Part model, mm, in its own coordinate system. Face numbers are marked on the shaded views. A direction names the side the tool comes from. Coordinates: 2 decimals unless noted, no trailing zeros. Write each loop counter-clockwise with the first axis right and the second up, starting at its lowest first coordinate (ties: lowest second). Pieces come first, ordered by that corner, then holes. Notation, with made-up numbers: (-18, 10.5) - (-5, 10.5) arc R13 cw to (-5, 21.5) - close; hole circle Ø6 at (-32.5, 52). An arc over 180 degrees is marked (long way). Use a Markdown table: item, result.
```python
from build123d import *

# Parameters (mm, degrees)
SKETCH1_W           = 30
SKETCH1_H           = 30
BOSS_EXTRUDE1_DEPTH = 2
SKETCH2_R           = 9
CUT_EXTRUDE1_DEPTH  = 22.307275753
FILLET1_R           = 15
SKETCH3_W           = 30
SKETCH3_H           = 2
BOSS_EXTRUDE2_DEPTH = 11
SKETCH4_R           = 1.5
CUT_EXTRUDE2_DEPTH  = 34.615472628
FILLET2_R           = 2


with BuildPart() as part:
    # Sketch1 → Boss-Extrude1 (new body)
    with BuildSketch(Plane.XY):
        Rectangle(SKETCH1_W, SKETCH1_H)
    extrude(amount=BOSS_EXTRUDE1_DEPTH)

    # Sketch2 → Cut-Extrude1 (cut, through all)
    with BuildSketch(Plane.XY.offset(2)):
        Circle(SKETCH2_R)
    extrude(amount=-CUT_EXTRUDE1_DEPTH, mode=Mode.SUBTRACT)

    # Fillet1
    fillet1_edges = [part.edges().sort_by_distance(p)[0] for p in [
        (-15, 15, 1),
        (15, 15, 1),
    ]]
    fillet(fillet1_edges, radius=FILLET1_R - 0.0001)  # a hair under: the kernel refuses the full size

    # Sketch3 → Boss-Extrude2 (add)
    with BuildSketch(Plane(origin=(0, 0, 0), x_dir=(-1, 0, 0), z_dir=(0, 0, -1))):
        with Locations((0, -14)):
            Rectangle(SKETCH3_W, SKETCH3_H)
    extrude(amount=BOSS_EXTRUDE2_DEPTH)

    # Sketch4 → Cut-Extrude2 (cut, through all)
    with BuildSketch(Plane(origin=(0, -13, 0), x_dir=(1, 0, 0), z_dir=(0, 1, 0))):
        with Locations(Location((0, 6, 0), (0, 0, 270))):
            Circle(SKETCH4_R)
    extrude(amount=-CUT_EXTRUDE2_DEPTH, mode=Mode.SUBTRACT)

    # Fillet2
    fillet2_edges = [part.edges().sort_by_distance(p)[0] for p in [
        (15, -14, -11),
        (-15, -14, -11),
        (0, -15, 2),
    ]]
    fillet(fillet2_edges, radius=FILLET2_R)


solid = part.part
```
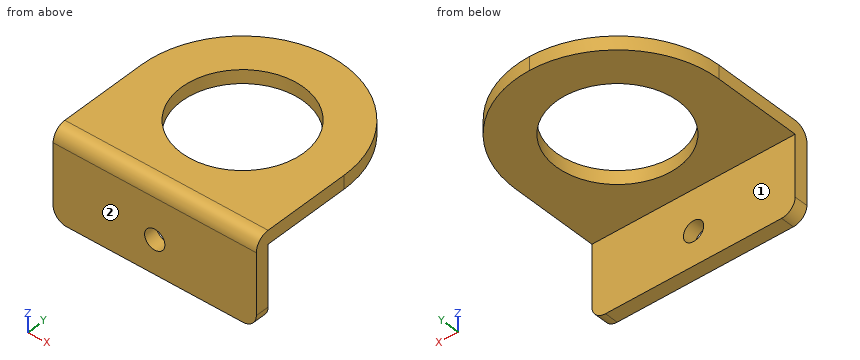
Item 1: Band-saw the part on A-A, the plane z = -6. Give the cut face in (x, y).
From the geometry:
| item | result |
|---|---|
| outline | (-15, -15) - (-1.5, -15) - (-1.5, -13) - (-15, -13) - close; (1.5, -15) - (15, -15) - (15, -13) - (1.5, -13) - close |
Item 2: Which spindle directions (+Z, -Z, +X, -X, +Y, -Y) get a long thin tool onto all of the face, cutting with end or side? Do the marked faces 1 and 2. Say none if no direction does.
From the geometry:
| item | result |
|---|---|
| face 1 | -Z, +X, -X, +Y |
| face 2 | +Z, -Z, +X, -X, -Y |
Item 3: Band-saw the part on B-B, the plane y = -4. Give the cut face in (x, z), then the cut area to 3 significant figures.
From the geometry:
| item | result |
|---|---|
| outline | (-15, 0) - (-8.06, 0) - (-8.06, 2) - (-15, 2) - close; (8.06, 0) - (15, 0) - (15, 2) - (8.06, 2) - close |
| area | 27.8 mm^2 |
Item 4: Drill centre lines: probe 1 along X at (y, z) = (-14.15, -6); probe 2 along Z at (x, y) = (10, 5); probe 3 along Y at (x, z) = (-7, -4.5). Where is each one in solid material? Low to high.
From the geometry:
| item | result |
|---|---|
| probe 1 | -15 to -1.5, 1.5 to 15 |
| probe 2 | 0 to 2 |
| probe 3 | -15 to -13 |
Item 5: Band-saw the part on C-C, the plane x = 5.5. Give the cut face in (y, z), then the cut area to 3 significant figures.
From the geometry:
| item | result |
|---|---|
| outline | (-15, -11) - (-13, -11) - (-13, 0) - (-7.12, 0) - (-7.12, 2) - (-13, 2) arc R2 ccw to (-15, 0) - close; (7.12, 0) - (13.96, 0) - (13.96, 2) - (7.12, 2) - close |
| area | 50.6 mm^2 |
Item 6: Drop flat-ended pins along their axis: P1, Ø1, axis at x = 7, z = -2.5, coming from the +Y side; P2, Ø6, axis at x = 3.5, z = 0, coming from the +Y side. Give the stop position or say it passes through.
From the geometry:
| item | result |
|---|---|
| P1 | y = -13 |
| P2 | y = 14.99 |
